Source: CAD feature listing. Evaluate the final solid. Frame: model axes, mm. Face numbers are marked on the shaded views. A direction names the side the tool comes from. Give positions to 0.01 mm unless a question says otherwise; leave off trailing zeros. Order: outer loops, then holes, each group sorted by start corner. A loop starts at its lowest first (then second) coordinate and runs counter-clockwise, first axis right, second up. Notation, with made-up numbers: M -24,-1.75 L -19,-1.75 A28 ccw -19,37.25 Z; hole C -31.5,-18 d9. An arc over 180 degrees is marked long. Answer in a Markdown table with one row per item. Add a question column.
(1) Mould query, pull axis Z, two halves, no side actions, for the marked faces 1, 2 and 3. Classes: pulls with the +Z half, pulls with the -Z half, needs draft (parallel to the pull), parting line crosses it, or undercut.
(2) Material intervals for line 1 along Z through (x, y) = (-7, 13) (3 decimals); line 2 along X through (y, z) = (23.5, 1); line 3 along X through (y, z) = (34, -10), sorted ascending.
(3) Section query C-C, the plane x = 20. Return loops of the section in (y, z) (3 decimals).
(4) Section query D-D, the plane y = 22. Return loops of the section in (x, z) (3 decimals).
(5) Pin query (flat end, axial travel): P1, Ø3, axis at x = 42, y = 10.5, coming from the +Z side; P2, Ø6, axis at x = 0.5, z = 9.5, coming from the +Y side; P3, Ø1.5, axis at x = -37, z = 9.5, coming from the +Y side; P4, Ø2, axis at x = 0.5, z = -15.5, coming from the +Y side. Return the tip coordinate at first contact, or that it passes through.
(6) Section query A-A, the plane y = 16. Return loops of the section in (x, z) (3 decimals).
(7) Set-up query: the marked faces 4 and 5. Return all of +Z, -Z, +X, -X, +Y, -Y with unobstructed straight access to the full face (end or side cutting, diameter ignored); none if empty.
(8) Section query B-B, the plane z = -3.5. Return loops of the section in (x, y) (3 decimals).
from build123d import *

# Parameters (mm, degrees)
SKETCH1_W           = 91.44
SKETCH1_H           = 45.72
BOSS_EXTRUDE1_DEPTH = 45
SKETCH2_W           = 65.278
SKETCH2_H           = 31.75
CUT_EXTRUDE1_DEPTH  = 40
SKETCH3_R           = 2.5
CUT_EXTRUDE2_DEPTH  = 25.4
FILLET1_R           = 5.08
FILLET3_R           = 1.27
FILLET4_R           = 0.508
SKETCH4_W           = 10.16
SKETCH4_H           = 6.35
CUT_EXTRUDE3_DEPTH  = 94.207899241


with BuildPart() as part:
    # Sketch1 → Boss-Extrude1 (new body)
    with BuildSketch(Plane(origin=(0, 0, 0), x_dir=(1, 0, 0), z_dir=(0, 1, 0))):
        Rectangle(SKETCH1_W, SKETCH1_H)
    extrude(amount=BOSS_EXTRUDE1_DEPTH)

    # Sketch2 → Cut-Extrude1 (cut)
    with BuildSketch(Plane(origin=(0, 45, 0), x_dir=(1, 0, 0), z_dir=(0, 1, 0))):
        Rectangle(SKETCH2_W, SKETCH2_H)
    extrude(amount=-CUT_EXTRUDE1_DEPTH, mode=Mode.SUBTRACT)

    # Sketch3 → Cut-Extrude2 (cut)
    with BuildSketch(Plane(origin=(0, 45, 0), x_dir=(1, 0, 0), z_dir=(0, 1, 0))):
        with Locations(Location((37.465, 8.509, 0), (0, 0, 270))):
            Circle(SKETCH3_R)
        with Locations(Location((37.465, -8.509, 0), (0, 0, 270))):
            Circle(SKETCH3_R)
        with Locations(Location((-37.465, -8.509, 0), (0, 0, 90))):
            Circle(SKETCH3_R)
        with Locations(Location((-37.465, 8.509, 0), (0, 0, 90))):
            Circle(SKETCH3_R)
    extrude(amount=-CUT_EXTRUDE2_DEPTH, mode=Mode.SUBTRACT)

    # Fillet1
    fillet1_edges = [part.edges().sort_by_distance(p)[0] for p in [
        (45.72, 22.5, 22.86),
        (-45.72, 22.5, 22.86),
        (-45.72, 22.5, -22.86),
        (45.72, 22.5, -22.86),
    ]]
    fillet(fillet1_edges, radius=FILLET1_R)

    # Fillet3
    fillet3_edges = [part.edges().sort_by_distance(p)[0] for p in [
        (32.639, 45, 0),
        (0, 45, -15.875),
        (-32.639, 45, 0),
        (0, 45, 15.875),
    ]]
    fillet(fillet3_edges, radius=FILLET3_R)

    # Fillet4
    fillet4_edges = [part.edges().sort_by_distance(p)[0] for p in [
        (-37.465, 45, -6.009),
        (-37.465, 45, 11.009),
        (37.465, 45, 6.009),
        (37.465, 45, -11.009),
    ]]
    fillet(fillet4_edges, radius=FILLET4_R)

    # Sketch4 → Cut-Extrude3 (cut, through all)
    with BuildSketch(Plane.ZY.offset(-32.639)):
        with Locations((0, 10.08)):
            Rectangle(SKETCH4_W, SKETCH4_H)
    extrude(amount=-CUT_EXTRUDE3_DEPTH, mode=Mode.SUBTRACT)


solid = part.part
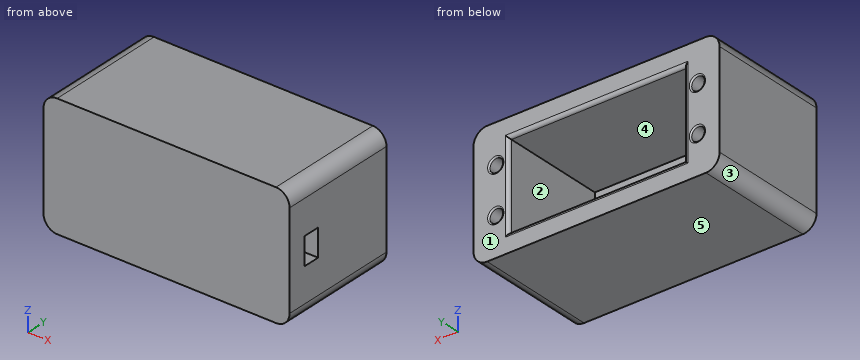
Values follow:
| question | item | result |
|---|---|---|
| 1 | face 1 | needs draft |
| 1 | face 2 | undercut |
| 1 | face 3 | pulls with the -Z half |
| 2 | line 1 | z = -22.86 to -15.875, 15.875 to 22.86 |
| 2 | line 2 | x = -45.72 to -32.64, 32.64 to 45.72 |
| 2 | line 3 | x = -45.72 to -39.47, -35.46 to -32.64, 32.64 to 35.46, 39.47 to 45.72 |
| 3 | outline | M 0,-22.86 L 45,-22.86 L 45,-17.145 A1.27 ccw 43.73,-15.875 L 5,-15.875 L 5,15.875 L 43.73,15.875 A1.27 ccw 45,17.145 L 45,22.86 L 0,22.86 Z |
| 4 | outline | M -45.72,-17.78 A5.08 ccw -40.64,-22.86 L 40.64,-22.86 A5.08 ccw 45.72,-17.78 L 45.72,17.78 A5.08 ccw 40.64,22.86 L -40.64,22.86 A5.08 ccw -45.72,17.78 Z; hole C -37.465,-8.509 d5; hole C -37.465,8.509 d5; hole M -32.639,-15.875 L 32.639,-15.875 L 32.639,15.875 L -32.639,15.875 Z; hole C 37.465,-8.509 d5; hole C 37.465,8.509 d5 |
| 5 | P1 | stops at z = 22.86 |
| 5 | P2 | stops at y = 5 |
| 5 | P3 | stops at y = 19.6 |
| 5 | P4 | stops at y = 44.82 |
| 6 | outline | M -45.72,-17.78 A5.08 ccw -40.64,-22.86 L 40.64,-22.86 A5.08 ccw 45.72,-17.78 L 45.72,17.78 A5.08 ccw 40.64,22.86 L -40.64,22.86 A5.08 ccw -45.72,17.78 Z; hole M -32.639,-15.875 L 32.639,-15.875 L 32.639,15.875 L -32.639,15.875 Z |
| 7 | face 4 | +Y |
| 7 | face 5 | -Z, +X, -X, +Y, -Y |
| 8 | outline | M -45.72,0 L 45.72,0 L 45.72,6.905 L 32.639,6.905 L 32.639,5 L -32.639,5 L -32.639,43.73 A1.27 ccw -33.909,45 L -45.72,45 Z; M 32.639,13.255 L 45.72,13.255 L 45.72,45 L 33.909,45 A1.27 ccw 32.639,43.73 Z |
